Check sheet for the modelled part. Datum: model origin and axes. Units: mm. A direction names the side the tool comes from. Give positions to 0.01 mm unless a question says otherwise; leave off trailing zeros. Write each loop counter-clockwise with the first axis right and the second up, starting at its lowest first coordinate (ties: lowest second). Pieces come first, ordered by that corner, then holes. Notation, with made-up numbers: M 69.25,2 L 111.25,2 A27 ccw 111.25,19 Z; hole C 54.25,84.5 d6. An arc over 180 degrees is marked long. Use CSV: the item, a comma, the result in double quotes. Start each with the question number.
1. Access from +Z, -Z, +X, -X, +Y, -Y to the whole of each face (thin tool, end or side, straight path). Record for faces 5 (the face through (0, -26, 0)), 6 (the face through (-12, 25.25, 1)), 7 (the face through (30, 25.25, 1)).
2. Mould release check, pull along X, two halves, no side actions. Record for faces 1 (the face through (23.5, 31, 1)), 2 (the face through (4.75, -25, -1)), 3 (the face through (-15.25, -25, -1)), 4 (the face through (-20, -26, 0)): +X half, -X half, draft (parallel to the pull), parting line (faces both ways), or undercut.
3. Cross-section at B-B, the plane z = 0.8. Enter the section's corners in (x, y), and give its area (3 significant figures).
4. Cross-section at C-C, the plane y = -11. Enter the section's corners in (x, z), and give its area (3 significant figures).
5. Depth check by flat-ended pin: P1, Ø1.2, axis at x = -0.5, y = -26.5, coming from the +Z side; P2, Ø1.6, axis at y = -25, z = -0.5, coming from the -X side; P3, Ø1, axis at x = 2, z = 0.5, coming from the +Y side; P4, Ø3, axis at x = 16, y = 32.75, coming from the -Z side. Enter the tip coordinate at first touch or a pass-through.
6. Scan lines: line 1 (X direction, y = -24.5, z = -0.15); line 2 (Y direction, x = 16, z = 0.85). Record each from-to range of solid material in increasing order.
from build123d import *

# Parameters (mm, degrees)
ESQUISSE1_R             = 2
BOSS_EXTRU_1_DEPTH      = 2
ESQUISSE2_W             = 9.5
ESQUISSE2_H             = 2
BOSS_EXTRU_2_DEPTH      = 2.5
CHANFREIN1_SIZE         = 2
ENL_V_MAT_EXTRU_2_REACH = 57.157
ESQUISSE4_W             = 6
ESQUISSE4_H             = 50.5
CONG_1_R                = 4


with BuildPart() as part:
    # Esquisse1 → Boss.-Extru.1 (new body)
    with BuildSketch(Plane.XY):
        with BuildLine():
            ThreePointArc((8.5, 32.75), (16, 40.25), (23.5, 32.75))
            Line((23.5, 32.75), (23.5, 25.25))
            Line((23.5, 25.25), (37.5, 25.25))
            Line((37.5, 25.25), (37.5, -25.25))
            Line((37.5, -25.25), (-37.5, -25.25))
            Line((-37.5, -25.25), (-37.5, 25.25))
            Line((-37.5, 25.25), (8.5, 25.25))
            Line((8.5, 25.25), (8.5, 32.75))
        make_face()
        with Locations((16, 32.75)):
            Circle(ESQUISSE1_R, mode=Mode.SUBTRACT)
    extrude(amount=BOSS_EXTRU_1_DEPTH)

    # Esquisse2 → Boss.-Extru.2 (add, symmetric)
    with BuildSketch(Plane.XZ.offset(25.25)):
        with Locations((0, -1)):
            Rectangle(ESQUISSE2_W, ESQUISSE2_H)
        with Locations((-20, -1)):
            Rectangle(ESQUISSE2_W, ESQUISSE2_H)
        with Locations((20, -1)):
            Rectangle(ESQUISSE2_W, ESQUISSE2_H)
    extrude(amount=BOSS_EXTRU_2_DEPTH, both=True)

    # Chanfrein1
    chanfrein1_edges = [part.edges().sort_by_distance(p)[0] for p in [
        (-20, -22.75, 0),
        (0, -22.75, 0),
        (20, -22.75, 0),
    ]]
    chamfer(chanfrein1_edges, length=CHANFREIN1_SIZE - 0.0001)  # a hair under: the kernel refuses the full size

    # Esquisse4 → Enlèv. mat.-Extru.2 (cut, up to next)
    with BuildSketch(Plane.XY.offset(2), mode=Mode.PRIVATE) as enl_v_mat_extru_2_sk1:
        with Locations((-34.5, 0)):
            Rectangle(ESQUISSE4_W, ESQUISSE4_H)
    enl_v_mat_extru_2_tool1 = extrude(enl_v_mat_extru_2_sk1.sketch, amount=-ENL_V_MAT_EXTRU_2_REACH, mode=Mode.PRIVATE) & part.part
    add(enl_v_mat_extru_2_tool1.solids().sort_by_distance((-34.5, 0, 2))[0], mode=Mode.SUBTRACT)

    # Congé1
    cong_1_edges = [part.edges().sort_by_distance(p)[0] for p in [
        (-31.5, 25.25, 1),
        (-31.5, -25.25, 1),
        (23.5, 25.25, 1),
        (37.5, 25.25, 1),
        (37.5, -25.25, 1),
        (8.5, 25.25, 1),
    ]]
    fillet(cong_1_edges, radius=CONG_1_R)


solid = part.part
Worked answers:
1,face 5,"+Z, +X, -X, -Y"
1,face 6,"+Z, -Z, -X, +Y"
1,face 7,"+Z, -Z, +X, +Y"
2,face 1,"+X half"
2,face 2,"undercut"
2,face 3,"undercut"
2,face 4,"draft"
3,outline,"M -31.5,-21.25 A4 ccw -27.5,-25.25 L 33.5,-25.25 A4 ccw 37.5,-21.25 L 37.5,21.25 A4 ccw 33.5,25.25 L 27.5,25.25 A4 cw 23.5,29.25 L 23.5,32.75 A7.5 ccw 8.5,32.75 L 8.5,29.25 A4 cw 4.5,25.25 L -27.5,25.25 A4 ccw -31.5,21.25 Z; hole C 16,32.75 d4"
3,area,"3,670 mm^2"
4,outline,"M -31.5,0 L 37.5,0 L 37.5,2 L -31.5,2 Z"
4,area,"138 mm^2"
5,P1,"stops at z = 0"
5,P2,"stops at x = -30"
5,P3,"stops at y = 25.25"
5,P4,"passes through"
6,line 1,"x = -24.75 to -15.25, -4.75 to 4.75, 15.25 to 24.75"
6,line 2,"y = -25.25 to 30.75, 34.75 to 40.25"
